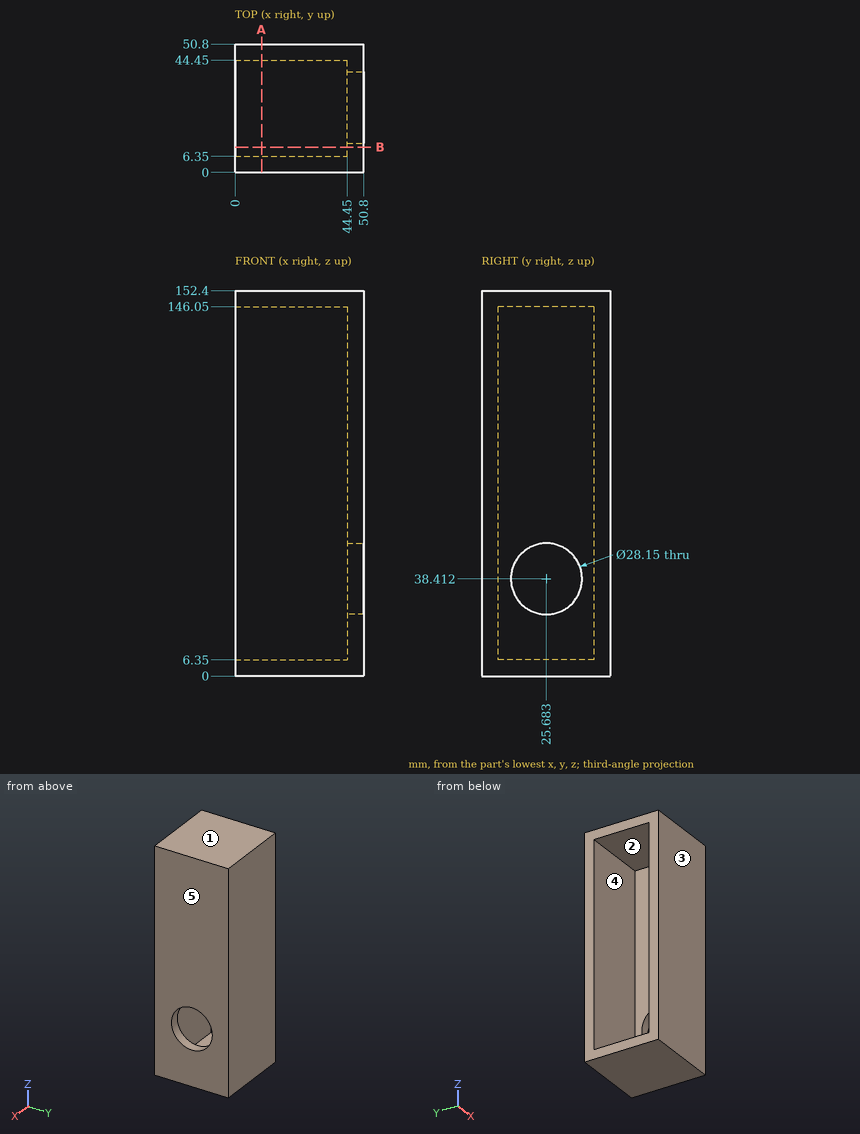
Here's the drawing with two shaded views (mm, measured from the low corner). I have some questions. A direction names the side the tool comes from. Coordinates: 2 decimals unless noted, no trailing zeros. Order: outer loops, then holes, each group sorted by start corner. A loop starts at its lowest first (then second) coordinate and runs counter-clockwise, first axis right, second up.
Q1. Suppose I cut it at A-A on x = 10.5. Please give me the cut outline in (y, z), and give its area (3 significant figures).
Q2. Will this pin go through, and if not, where does the flat tip stop? pin 1 (5 mm diameter, centred on y = 23.5, z = 75, fed in from -X).
Q3. Thinking about a two-plate mould opening in Z: for the marked faces 1, 2 and 3, which applies, released by +Z, released by -Z, zero draft, split by the parting line, or undercut?
Q4. Which directions (+Z, -Z, +X, -X, +Y, -Y) give clear straight access to the entire face, cutting with the end or side of a thin tool? Please do the marked faces 4 and 5.
Q5. Please list where these lines run through material, in increasing order: L1, parallel to Z at x = 11.5, y = 7.5; L2, parallel to Y at x = 2, z = 29.5.
Q6. Suppose I cut it at B-B on y = 10. Please give me the cut outline in (x, z), and give its area (3 significant figures).
Answer:
1. outline: (0, 0) - (50.8, 0) - (50.8, 152.4) - (0, 152.4) - close; hole (6.35, 6.35) - (44.45, 6.35) - (44.45, 146.05) - (6.35, 146.05) - close
1. area: 2,420 mm2
2. pin 1: stops at x = 44.45
3. face 1: released by +Z
3. face 2: undercut
3. face 3: zero draft
4. face 4: -X
4. face 5: +Z, -Z, +X, +Y, -Y
5. L1: z = 0 to 6.35, 146.05 to 152.4
5. L2: y = 0 to 6.35, 44.45 to 50.8
6. outline: (0, 0) - (50.8, 0) - (50.8, 152.4) - (0, 152.4) - (0, 146.05) - (44.45, 146.05) - (44.45, 6.35) - (0, 6.35) - close
6. area: 1,530 mm2
